Autodesk Inventor part; units mm, degrees
ref_plane "Work Plane2" through (3.35, 0, 0) normal (0, 0, -1) x (1, 0, 0)
ref_plane "YZ Plane" through (0, 0, 0) normal (1, 0, 0) x (0, 1, 0)
ref_plane "XZ Plane" through (0, 0, 0) normal (0, 1, 0) x (-1, 0, 0)
sketch "Sketch1" plane through (0, 0, 0) normal (0, 0, 1) x (1, 0, 0)
  line L0 (3.2, 0) -> (16, 0)
  line L1 (16, 0) -> (16, 2.5)
  line L2 (16, 2.5) -> (4.3, 2.5)
  line L3 (4.3, 2.5) -> (3.8092, 2.2546)
  line L4 (3.8092, 2.2546) -> (2.7, 2.2546)
  line L5 (0, 4.65) -> (0, 2.6)
  line L6 (0, 2.6) -> (2.4732, 1.3669)
  line L7 (2.4732, 1.3669) -> (3.2, 0)
  line L8 (-3.2, 0) -> (19.2, 0)
  line L9 (0, -0.93) -> (0, 5.58)
  line L10 (0, 4.65) -> (0.3046, 4.65)
  line L11 (0.3046, 4.65) -> (2.7, 2.2546)
  line L12 (4.3, 2.5) -> (2.4546, 2.5) construction
  dimension "d1" = 11.7
  dimension "d2" = 5
  dimension "d3" = 4.5092
  dimension "d4" = 5.2
  dimension "d5" = 26.5
  dimension "d6" = 62
  dimension "d7" = 3.2
  dimension "d8" = 0.4908
  dimension "d12" = 9.3
  dimension "d13" = 45
  dimension "d15" = 16
  dimension "d24" = 2.7
revolve "Body" add sketch "Sketch1" angle 360 about axis through (3.2, 0, 0) along (1, 0, 0) contours L7 L6 L5 L10 L11 L4 L3 L2 L1 L0
sketch "Sketch2" plane through (0, 0, 0) normal (-1, 0, 0) x (0, 0, 1)
  line L0 (0, 2.6) -> (0, 0) construction
  line L1 (0, 0) -> (2.6, 0) construction
  arc A0 (0.78, 0) -> (0, 0.78) centre (0, 0) ccw construction
  arc A1 (0.91, 0) -> (0, 0.91) centre (0, 0) ccw construction
  arc A2 (2.579, 0.33) -> (0.33, 2.579) centre (0, 0) ccw
  line L2 (0, 0) -> (1.8385, 1.8385) construction
  line L3 (0.33, 2.579) -> (0.4413, 0.7958)
  line L4 (2.579, 0.33) -> (0.7958, 0.4413)
  arc A3 (0.33, 2.579) -> (0, 2.6) centre (0, 0) ccw
  arc A4 (2.6, 0) -> (2.579, 0.33) centre (0, 0) ccw
  line L5 (0, -6.51) -> (0, 6.51)
  line L6 (-6.51, 0) -> (6.51, 0)
  arc A5 (0.33, -2.579) -> (2.579, -0.33) centre (0, 0) ccw
  line L7 (0.33, -2.579) -> (0.4413, -0.7958)
  line L8 (2.579, -0.33) -> (0.7958, -0.4413)
  arc A6 (0, -2.6) -> (0.33, -2.579) centre (0, 0) ccw
  arc A7 (2.579, -0.33) -> (2.6, 0) centre (0, 0) ccw
  arc A8 (-0.33, 2.579) -> (-2.579, 0.33) centre (0, 0) ccw
  line L9 (-0.33, 2.579) -> (-0.4413, 0.7958)
  line L10 (-2.579, 0.33) -> (-0.7958, 0.4413)
  arc A9 (0, 2.6) -> (-0.33, 2.579) centre (0, 0) ccw
  arc A10 (-2.579, 0.33) -> (-2.6, 0) centre (0, 0) ccw
  arc A11 (-0.33, -2.579) -> (0, -2.6) centre (0, 0) ccw
  arc A12 (-2.579, -0.33) -> (-0.33, -2.579) centre (0, 0) ccw
  arc A13 (-2.6, 0) -> (-2.579, -0.33) centre (0, 0) ccw
  line L11 (-2.579, -0.33) -> (-0.7958, -0.4413)
  line L12 (-0.33, -2.579) -> (-0.4413, -0.7958)
  arc A14 (0.4413, 0.7958) -> (0.7958, 0.4413) centre (0.8194, 0.8194) ccw
  arc A15 (0.7958, -0.4413) -> (0.4413, -0.7958) centre (0.8194, -0.8194) ccw
  arc A16 (-0.7958, 0.4413) -> (-0.4413, 0.7958) centre (-0.8194, 0.8194) ccw
  arc A17 (-0.4413, -0.7958) -> (-0.7958, -0.4413) centre (-0.8194, -0.8194) ccw
  point P0 (1.8385, -1.8385)
  point P1 (-1.8385, 1.8385)
  point P2 (-1.8385, -1.8385)
  dimension "d17" = 1.56
  dimension "d18" = 1.82
  dimension "d19" = 5.2
  dimension "d20" = 45
  dimension "d21" = 0.33
extrude "Slot" add sketch "Sketch2" against normal up to next draft 5 contours L4 A14 L3 A2 | A5 L7 A15 L8 | L9 A16 L10 A8 | A12 L11 A17 L12
fillet "Fillet1" radius 0.132 4 edges at (0, 2.6, 0) (0, 0, -2.6) (0, -2.6, 0) (0, 0, 2.6)
thread "Thread"
chamfer "Chamfer1" distance 0.4908 distance2 0.2454 1 edges at (16, -2.5, 0) measured on face at (16, 0.2278, 0.5045)
ref_plane "Work Plane2" through (3.35, 0, 0) normal (0, 0, -1) x (1, 0, 0)
equation "\"d17\" = 0.3 * SDM"
equation "\"d18\" = 0.35 * SDM"
equation "\"d19\" = SDM"
equation "\"d21\" = 0.5 * SBR"
equation "\"d1\" = GEL"
equation "\"d2\" = GD"
equation "\"d3\" = BDM"
equation "\"d4\" = SDM"
equation "\"d7\" = INTI"
equation "\"d8\" = GAL"
equation "\"d12\" = KOD"
equation "\"d13\" = 0.5 * SEWI"
equation "\"d15\" = NLG"
equation "\"d24\" = KOH"
equation "\"d23\" = 0.2 * SBR"
equation "\"d10\" = GEL"
equation "\"d25\" = -0.5 * SPD + 0.5 * GD"
equation "\"d26\" = 0.5 * GAL"
equation "\"NLG\" = 16"
equation "\"GEL\" = 11.7"
equation "\"GAL\" = 0.61345 * PTC"
equation "\"SPD\" = NND - 1.2269 * PTC"
equation "\"KOD\" = 9.3"
equation "\"KOH\" = 2.7"
equation "\"SBR\" = 0.66"
equation "\"INTI\" = 3.2"
equation "\"SDM\" = 5.2"
equation "\"GD\" = NND"
equation "\"BDM\" = NND - GAL"
equation "\"SEWI\" = 90deg"
equation "\"d9\" = SDM"
equation "\"GUL\" = 0.61345 * PTC"
equation "\"TOA\" = 30deg"
equation "\"EPV\" = 5.2"
equation "\"THREADDIA\" = 5"
equation "\"PTC\" = 0.8"
equation "\"NND\" = 5"
equation "\"GD1\" = THREADDIA - 1.2269 * PTC"
properties part number "ISO 7046-1 - M5 x 16 - 4.8 - H" material "Steel"
Check sheet for the modelled part. Datum: model origin and axes. Units: mm. A direction names the side the tool comes from. Give positions to 0.01 mm unless a question says otherwise; leave off trailing zeros. Order: outer loops, then holes, each group sorted by start corner. A loop starts at its lowest first (then second) coordinate and runs counter-clockwise, first axis right, second up. Notation, with made-up numbers: M 20.5,25.25 L 79.5,25.25 A30 ccw 79.5,60.25 Z; hole C 26.25,65 d3. An arc over 180 degrees is marked long. Answer in a Markdown table with one row per item.
1) Access from +Z, -Z, +X, -X, +Y, -Y to the whole of each face (thin tool, end or side, straight path). Record for faces 1 (the cylindrical face through (3.25, 2.15, -0.68)), 2 (the flat face through (1.058, -0.316, 1.321)), 3 (the cylindrical face through (0.154, 2.5, 3.921)).
Filled sheet:
| item | result |
|---|---|
| face 1 | none |
| face 2 | -X |
| face 3 | +X, -X |
2) Gauge pin test, flat ends, axial feed: P1, Ø1, axis at x = 3.5, z = -3.5, coming from the -Y side; P2, Ø3, axis at x = 10.5, z = 2, coming from the +Y side; P3, Ø2, axis at x = 8, z = 2.5, coming from the -Y side. Record the tip position at first contact, or that the pin passes through.
Filled sheet:
| item | result |
|---|---|
| P1 | passes through |
| P2 | stops at y = 2.45 |
| P3 | stops at y = -2 |
3) Thickness scan on L1, parallel to Z at x = 2, y = -1; L2, parallel to X at y = 2.25, z = 0.5; L3, parallel to Y at x = 2, z = -0.5. Record the ranges inside material, lowest first. Write a range as [from, to].
Filled sheet:
| item | result |
|---|---|
| L1 | z = [-2.78, -0.25], [0.25, 2.78] |
| L2 | x = [0, 2.65], [3.91, 15.85] |
| L3 | y = [-2.91, -0.37], [0.37, 2.91] |
4) Cross-section at A-A, the plane x = 12.5. Enter the section's corners in (y, z), plus the area to 3 significant figures.
Filled sheet:
| item | result |
|---|---|
| outline | C 0,0 d5 |
| area | 19.6 mm2 |
5) Release check for a two-part mould opening along Z. For faces 4 (the flat face through (1.058, 1.321, 0.316)), 5 (the flat face through (16, 0, 0)), 6 (the cylindrical face through (9.95, -0.54, 2.44)) record: +Z half, -Z half, draft (parallel to the pull), parting line (faces both ways), or undercut.
Filled sheet:
| item | result |
|---|---|
| face 4 | undercut |
| face 5 | draft |
| face 6 | parting line |
